Here's how the part is built. I have some questions about the finished solid (model axes, mm). A direction names the side the tool comes from. Coordinates: 2 decimals unless noted, no trailing zeros. Write each loop counter-clockwise with the first axis right and the second up, starting at its lowest first coordinate (ties: lowest second). Pieces come first, ordered by that corner, then holes. Notation, with made-up numbers: M 68.25,16 L 77.25,16 A33 cw 77.25,47 Z; hole C -25.75,37.5 d10. An arc over 180 degrees is marked long. Write each question's results on one line, items separated by ' | '. Start each with the question number.
from build123d import *

# Parameters (mm, degrees)
SKETCH_1_R               = 22.5
EXTRUDE_1_DEPTH          = 10.5
SKETCH_2_R               = 15
EXTRUDE_2_DEPTH          = 5
SKETCH_3_R               = 1.5
CUT_EXTRUDE_1_DEPTH      = 5
SKETCH_5_R               = 1.5
CUT_EXTRUDE_2_DEPTH      = 34.507461856
CUT_EXTRUDE_6_DEPTH      = 3
PATTERN_CIRCULAR_1_COUNT = 12


with BuildPart() as part:
    # 草图1 → 凸台-拉伸1 (new body)
    with BuildSketch(Plane.XY):
        with Locations(Location((0, 0, 0), (0, 0, 180))):
            Circle(SKETCH_1_R)
    extrude(amount=EXTRUDE_1_DEPTH)

    # 草图2 → 凸台-拉伸2 (add)
    with BuildSketch(Plane.XY.offset(10.5)):
        Circle(SKETCH_2_R)
    extrude(amount=EXTRUDE_2_DEPTH)

    # 草图3 → 切除-拉伸1 (cut)
    with BuildSketch(Plane.XY.offset(10.5)):
        with Locations((0, 18.5)):
            Circle(SKETCH_3_R)
    cut_extrude_1 = extrude(amount=-CUT_EXTRUDE_1_DEPTH, mode=Mode.SUBTRACT)

    # 草图5 → 切除-拉伸2 (cut, through all)
    with BuildSketch(Plane.XY.offset(10.5)):
        with Locations((0, 18.5)):
            Circle(SKETCH_5_R)
    cut_extrude_2 = extrude(amount=-CUT_EXTRUDE_2_DEPTH, mode=Mode.SUBTRACT)

    # 草图9 → 切除-拉伸6 (cut)
    with BuildSketch(Plane(origin=(0, 0, 0), x_dir=(-1, 0, 0), z_dir=(0, 0, -1))):
        Polygon((1.313991975, 21.705218415), (-2.118804585, 21.240559639), (-3.43279656, 18.035341223), (-1.313991975, 15.294781585), (2.118804585, 15.759440361), (3.43279656, 18.964658777), align=None)
    cut_extrude_6 = extrude(amount=-CUT_EXTRUDE_6_DEPTH, mode=Mode.SUBTRACT)

    # 阵列(圆周)1: 切除-拉伸1, 切除-拉伸2, 切除-拉伸6 ×12 about axis
    pattern_circular_1_axis = Axis((0, 0, 0), (0, 0, 1))
    add([cut_extrude_1.rotate(pattern_circular_1_axis, i * 360 / PATTERN_CIRCULAR_1_COUNT) for i in range(1, PATTERN_CIRCULAR_1_COUNT)], mode=Mode.SUBTRACT)
    add([cut_extrude_2.rotate(pattern_circular_1_axis, i * 360 / PATTERN_CIRCULAR_1_COUNT) for i in range(1, PATTERN_CIRCULAR_1_COUNT)], mode=Mode.SUBTRACT)
    add([cut_extrude_6.rotate(pattern_circular_1_axis, i * 360 / PATTERN_CIRCULAR_1_COUNT) for i in range(1, PATTERN_CIRCULAR_1_COUNT)], mode=Mode.SUBTRACT)


solid = part.part
1) For pin 1 Ø4 at (y, z) = (10.5, 7.5) entering from -X; pin 2 Ø8 at (y, z) = (-8.5, 3.5) entering from +X; pin 3 Ø5 at (x, y) = (16.02, -9.25) entering from +Z, each with a flat end and sliding along its axis, tell me the tip position at first contact or that it passes through.
2) For faces 3 (the flat face through (-7.434, -13.633, 1.479)), 4 (the cylindrical face through (-20, 0, 7)), which set-ups out of +Z, -Z, +X, -X, +Y, -Y let a thin tool reach every point of the face, with its end or its side?
3) I want a section at A-A, the plane y = 0. Write out the boundary of the cut face in (x, z).
4) I want a section at C-C, the plane z = 6. Give the number of separate pieces and of enclosed holes in the cut face, then the cut area to 3 significant figures.
5) We'd pull the mould along X, two halves only. Please class faces 1 (the cylindrical face through (-10.382, 19.961, 5.176)), 2 (the flat face through (15, -11, 3)): pulls with the +X half, pulls with the -X half, needs draft (parallel to the pull), parting line crosses it, or undercut.
6) Please list where these lines run through material, in increasing order: line 1 (Y direction, x = 1, z = 5.25); line 2 (Y direction, x = -9.5, z = 9.5). Write a range as [from, to].
7) I want a section at D-D, the plane x = -5. Write out the boundary of the cut face in (y, z).
Output:
1) pin 1: stops at x = -20.83 | pin 2: stops at x = 22.05 | pin 3: stops at z = 10.5
2) face 3: -Z | face 4: +Z, -Z
3) outline: M -22.5,0 L -21.53,0 L -21.53,3 L -20,3 L -20,10.5 L -22.5,10.5 Z; M -17,3 L -15.47,3 L -15.47,0 L 15.47,0 L 15.47,3 L 17,3 L 17,10.5 L 15,10.5 L 15,15.5 L -15,15.5 L -15,10.5 L -17,10.5 Z; M 20,3 L 21.53,3 L 21.53,0 L 22.5,0 L 22.5,10.5 L 20,10.5 Z
4) separate pieces: 1 | enclosed holes: 12 | area: 1,510 mm2
5) face 1: parting line crosses it | face 2: undercut
6) line 1: y = [-22.48, -19.62], [-17.38, 17.38], [19.62, 22.48] | line 2: y = [-20.4, -17.5], [-14.54, 14.54], [17.5, 20.4]
7) outline: M -21.94,0 L 21.94,0 L 21.94,10.5 L 14.14,10.5 L 14.14,15.5 L -14.14,15.5 L -14.14,10.5 L -21.94,10.5 Z
